Geometry check sheet. Reference: the model listing, model coordinates, mm. A direction names the side the tool comes from. Coordinates: 2 decimals unless noted, no trailing zeros. Write each loop counter-clockwise with the first axis right and the second up, starting at its lowest first coordinate (ties: lowest second). Pieces come first, ordered by that corner, then holes. Notation, with made-up numbers: (35, 38.5) -> (87, 38.5) arc R13 cw to (87, 42.5) -> close; hole circle Ø4 at (77.25, -16). An arc over 180 degrees is marked (long way). One line per question, with ' | ' between items.
```python
from build123d import *

# Parameters (mm, degrees)
SKETCH_1_W          = 68
SKETCH_1_H          = 44
EXTRUDE_1_DEPTH     = 2
SKETCH_2_R          = 2.5
EXTRUDE_2_DEPTH     = 10
SKETCH_4_R          = 1.55
CUT_EXTRUDE_1_DEPTH = 42.713307229
FILLET_1_R          = 2


with BuildPart() as part:
    # 草图1 → 凸台-拉伸1 (new body)
    with BuildSketch(Plane(origin=(0, 0, 0), x_dir=(1, 0, 0), z_dir=(0, 1, 0))):
        Rectangle(SKETCH_1_W, SKETCH_1_H)
    extrude(amount=EXTRUDE_1_DEPTH)

    # 草图2 → 凸台-拉伸2 (add)
    with BuildSketch(Plane(origin=(0, 2, 0), x_dir=(1, 0, 0), z_dir=(0, 1, 0))):
        with Locations(Location((-18.362121931, 0, 0), (0, 0, 90))):
            Circle(SKETCH_2_R)
        with Locations(Location((-8.514245581, 0, 0), (0, 0, 90))):
            Circle(SKETCH_2_R)
        with Locations(Location((8.514245581, 0, 0), (0, 0, 90))):
            Circle(SKETCH_2_R)
        with Locations(Location((18.362121931, 0, 0), (0, 0, 90))):
            Circle(SKETCH_2_R)
    extrude(amount=EXTRUDE_2_DEPTH)

    # 草图4 → 切除-拉伸1 (cut, through all)
    with BuildSketch(Plane(origin=(0, 2, 0), x_dir=(1, 0, 0), z_dir=(0, 1, 0))):
        with Locations(Location((-30.75, 18.75, 0), (0, 0, 270))):
            Circle(SKETCH_4_R)
        with Locations(Location((-30.75, -18.75, 0), (0, 0, 90))):
            Circle(SKETCH_4_R)
        with Locations(Location((30.75, -18.75, 0), (0, 0, 270))):
            Circle(SKETCH_4_R)
        with Locations(Location((30.75, 18.75, 0), (0, 0, 90))):
            Circle(SKETCH_4_R)
    extrude(amount=-CUT_EXTRUDE_1_DEPTH, mode=Mode.SUBTRACT)

    # 圆角1
    fillet_1_edges = [part.edges().sort_by_distance(p)[0] for p in [
        (34, 1, 22),
        (-34, 1, 22),
        (-34, 1, -22),
        (34, 1, -22),
    ]]
    fillet(fillet_1_edges, radius=FILLET_1_R)


solid = part.part
```
(1) Material ranges on line 1 (X direction, y = 0.6, z = -18.75); line 2 (Y direction, x = 0.5, z = -1.5); line 3 (Z direction, x = -10.5, y = 9), recorded low to high.
Answers below:
line 1: x = -34 to -32.3, -29.2 to 29.2, 32.3 to 34 | line 2: y = 0 to 2 | line 3: z = -1.52 to 1.52
(2) Cross-section at D-D (y = 5.75). Record the cut outline in (x, z), plus the area to 3 significant figures.
Answers below:
outline: circle Ø5 at (-18.36, 0); circle Ø5 at (-8.51, 0); circle Ø5 at (8.51, 0); circle Ø5 at (18.36, 0) | area: 78.5 mm²
(3) Depth check by flat-ended pin: P1, Ø1.5, axis at y = 3.5, z = 2.5, coming from the -X side; P2, Ø3, axis at x = 30.75, z = -18.75, coming from the +Y side; P3, Ø5, axis at x = 30.75, z = 18.75, coming from the +Y side. Enter the tip coordinate at first touch or a pass-through.
Answers below:
P1: stops at x = -20.15 | P2: passes through | P3: stops at y = 2
(4) Draft check along Z on faces 3 (the face through (10.732, 6.93, -1.154)), 4 (the face through (32.287, 1.014, 18.548)), 5 (the face through (0, 1, -22)), 6 (the face through (-29.44, 1.01, -17.92)). Enter one of: pulls with the +Z half, pulls with the -Z half, needs draft (parallel to the pull), parting line crosses it, or undercut.
Answers below:
face 3: parting line crosses it | face 4: undercut | face 5: pulls with the -Z half | face 6: undercut
(5) Cross-section at A-A (z = -18.75). Record the cut outline in (x, y).
Answers below:
outline: (-34, 0) -> (-32.3, 0) -> (-32.3, 2) -> (-34, 2) -> close; (-29.2, 0) -> (29.2, 0) -> (29.2, 2) -> (-29.2, 2) -> close; (32.3, 0) -> (34, 0) -> (34, 2) -> (32.3, 2) -> close
(6) Tool access check on faces 1 (the face through (-10.993, 6.93, 0.325)), 2 (the face through (34, 1, 0)). Record the directions out of +Z, -Z, +X, -X, +Y, -Y that give a thin tool (end or side, any length) a straight path to the whole face; none if there is none.
Answers below:
face 1: +Y | face 2: +Z, -Z, +X, +Y, -Y
(7) Cross-section at B-B (x = -30.75). Record the cut outline in (y, z), plus the area to 3 significant figures.
Answers below:
outline: (0, -22) -> (2, -22) -> (2, -20.3) -> (0, -20.3) -> close; (0, -17.2) -> (2, -17.2) -> (2, 17.2) -> (0, 17.2) -> close; (0, 20.3) -> (2, 20.3) -> (2, 22) -> (0, 22) -> close | area: 75.6 mm²
(8) Cross-section at C-C (z = 0). Record the cut outline in (x, y), plus the area to 3 significant figures.
Answers below:
outline: (-34, 0) -> (34, 0) -> (34, 2) -> (20.86, 2) -> (20.86, 12) -> (15.86, 12) -> (15.86, 2) -> (11.01, 2) -> (11.01, 12) -> (6.01, 12) -> (6.01, 2) -> (-6.01, 2) -> (-6.01, 12) -> (-11.01, 12) -> (-11.01, 2) -> (-15.86, 2) -> (-15.86, 12) -> (-20.86, 12) -> (-20.86, 2) -> (-34, 2) -> close | area: 336 mm²
